For this review, take the finished solid that the model builds, in its own axes (mm). Round coordinates to 2 decimals unless told otherwise and drop trailing zeros. Write each loop counter-clockwise with the first axis right and the second up, starting at its lowest first coordinate (ties: lowest second). Pieces come first, ordered by that corner, then holes. Notation, with made-up numbers: (33.25, 59) -> (78.25, 59) arc R18 ccw to (78.25, 73) -> close; hole circle Ø7 at (49.5, -12). An arc over 180 degrees is marked (long way). Write each question's results on one line, items separated by ' | '. Start each with the question number.
Item 1: Add section A-A (z = -1.3). State the section outline as (x, y) points, plus the area to 3 significant figures.
Item 2: Clearance check with a flat-ended pin moving along its axis: pin 1 (2 mm diameter, centred on x = 1.5, z = -2.5, fed in from +Y). State where the tip first meets the part, or that it passes through.
Item 3: To check wall thickness, follow line 1 along X through (y, z) = (-1.5, -1.8); line 2 along Y through (x, z) = (-1.5, -1.15); line 3 along Y through (x, z) = (1, -3.1). State the ranges of each line that lie inside material, in increasing order.
Item 4: The part is to be moulded in two halves that separate along X. For faces 1 (the flat face through (3.5, 0, -2)), 2 (the conical face through (-3.149, 1.808, -3.724)), 3 (the conical face through (-0.009, 3.632, -3.724)), 4 (the cylindrical face through (-1.216, 1.115, -1.91)), say which applies: +X half, -X half, draft (parallel to the pull), parting line (faces both ways), or undercut.
from build123d import *

# Parameters (mm, degrees)
BASENUT_START = -3.8
BASENUTSKE_R  = 1.65
BASENUT_DEPTH = 3.8


# Read off the part's stored shape, not the designer's step: ThreadSchematic
with BuildPart() as part:
    # BaseNutSke → BaseNut (new body)
    with BuildSketch(Plane.XY.offset(BASENUT_START)):
        Polygon((3.5, 2.020725942), (3.5, -2.020725942), (0, -4.041451884), (-3.5, -2.020725942), (-3.5, 2.020725942), (0, 4.041451884), align=None)
        Circle(BASENUTSKE_R, mode=Mode.SUBTRACT)
    extrude(amount=BASENUT_DEPTH)

    # Sketch5 (on Front Plane) → EndChamfer (revolve, cut)
    with BuildSketch(Plane.XY):
        Polygon((3.7746, 2), (3.505020098, 1.615), (3.8254, 1.615), (3.8254, 2), align=None)
    revolve(axis=Axis((3.7746, 2, 0), (-0.5735764363510478, -0.8191520442889905, 0)), mode=Mode.SUBTRACT)

    # Sketch3 → Double-Chamfer (revolve, cut)
    with BuildSketch(Plane(origin=(0, 0, 0), x_dir=(0, 0, -1), z_dir=(1, 0, 0))):
        Polygon((3.8, 3.5), (3.487392609, 4.041451884), (3.487392609, 14.041451884), (13.8, 14.041451884), (13.8, 3.5), align=None)
        Polygon((0.312607391, 14.041451884), (-10, 14.041451884), (-10, 3.5), (0, 3.5), (0.312607391, 4.041451884), align=None)
    revolve(axis=Axis((0, 0, 0), (0, 0, -1)), mode=Mode.SUBTRACT)

    # ThreadSchematic outline → ThreadSchematic (revolve, cut)
    with BuildSketch(Plane.XZ):
        Polygon((1.65, 0), (1.65, -0.245072638), (2, 0), align=None)
        Polygon((2, -3.7746), (1.65, -3.529527362), (1.65, -3.8), (2, -3.8), align=None)
    revolve(axis=Axis((0, 0, 0), (0, 0, 1)), mode=Mode.SUBTRACT)


solid = part.part
Responses:
1) outline: (-3.5, -2.02) -> (0, -4.04) -> (3.5, -2.02) -> (3.5, 2.02) -> (0, 4.04) -> (-3.5, 2.02) -> close; hole circle Ø3.3 at (0, 0) | area: 33.9 mm^2
2) pin 1: stops at y = 3.75
3) line 1: x = -3.5 to -0.69, 0.69 to 3.5 | line 2: y = -3.18 to -0.69, 0.69 to 3.18 | line 3: y = -3.46 to -1.31, 1.31 to 3.46
4) face 1: +X half | face 2: -X half | face 3: parting line | face 4: undercut
